Autodesk Inventor part; units mm, degrees
ref_plane "YZ Plane" through (0, 0, 0) normal (1, 0, 0) x (0, 1, 0)
ref_plane "XZ Plane" through (0, 0, 0) normal (0, 1, 0) x (-1, 0, 0)
ref_plane "XY Plane" through (0, 0, 0) normal (0, 0, 1) x (1, 0, 0)
sketch "Sketch1" plane through (0, 0, 0) normal (0, 0, 1) x (1, 0, 0)
  line L0 (21.4217, 22.24) -> (21.4217, 19.24)
  line L1 (21.4217, 22.24) -> (37.8228, 22.24)
  line L2 (21.4217, 19.24) -> (40.8228, 19.24)
  line L3 (40.8228, 27.84) -> (37.8228, 27.84)
  line L4 (37.8228, 27.84) -> (37.8228, 22.24)
  line L5 (40.8228, 27.84) -> (40.8228, 19.24)
  point P0 (0, 0)
extrude "Extrusion1" add sketch "Sketch1" along normal blind 40
sketch "Sketch2" plane through (40.8228, 19.24, 0) normal (1, 0, 0) x (0, 0, -1)
  line L0 (-40, 8.6) -> (-40, 0)
  line L1 (0, 8.6) -> (-40, 8.6)
  circle A0 centre (-37, 5.8) radius 1.35
  circle A1 centre (-20, 5.8) radius 1.35
  circle A2 centre (-3, 5.8) radius 1.35
  point P0 (0, -19.24)
  dimension "d2" = 2.7
  dimension "d3" = 2.7
  dimension "d4" = 2.8
  dimension "d5" = 2.8
  dimension "d6" = 17
  dimension "d7" = 2.7
  dimension "d8" = 17
  dimension "d9" = 3
extrude "Extrusion2" cut sketch "Sketch2" against normal through all
sketch "Sketch3" plane through (21.4217, 22.24, 0) normal (0, 1, 0) x (1, 0, 0)
  line L0 (16.4011, 0) -> (0, 0)
  line L1 (0, 0) -> (0, -40)
  circle A0 centre (2.8, -3) radius 1.35
  circle A1 centre (2.8, -20) radius 1.35
  circle A2 centre (2.8, -37) radius 1.35
  point P0 (-21.4217, 0)
  dimension "d12" = 2.7
  dimension "d13" = 3
  dimension "d14" = 2.8
  dimension "d15" = 2.7
  dimension "d16" = 2.7
  dimension "d17" = 17
  dimension "d18" = 17
extrude "Extrusion3" cut sketch "Sketch3" against normal through all
properties part number "Groin" material "Aluminum-6061"
Work out the finished part from the listing and answer in its coordinate system (mm). Give positions to 0.01 mm unless a question says otherwise; leave off trailing zeros. Loops run counter-clockwise (first coordinate to the right, second up) from the corner with the lowest first, then second, coordinate; pieces in that order, holes last. Notation, with made-up numbers: (49.25, -8) - (85.25, -8) arc R14 ccw to (85.25, 17) - close; hole circle Ø7 at (46.25, 65.5). An arc over 180 degrees is marked (long way). One line per question, with ' | ' between items.
(1) Each of these flat-tipped pins is pushed along its axis until it touches: pin 1 Ø8 at (x, z) = (30, 17) entering from +Y; pin 2 Ø1.7 at (y, z) = (25, 22) entering from -X. Where does it stop, or does it pass through?
Recorded:
pin 1: stops at y = 22.24 | pin 2: stops at x = 37.82
(2) The part is cut by section C-C (y = 25.04). Write down the section's boundary in (x, z), then the cut area to 3 significant figures.
Recorded:
outline: (37.82, 0) - (40.82, 0) - (40.82, 1.65) - (37.82, 1.65) - close; (37.82, 4.35) - (40.82, 4.35) - (40.82, 18.65) - (37.82, 18.65) - close; (37.82, 21.35) - (40.82, 21.35) - (40.82, 35.65) - (37.82, 35.65) - close; (37.82, 38.35) - (40.82, 38.35) - (40.82, 40) - (37.82, 40) - close | area: 95.7 mm²
(3) Straight lines are drawn through the part: probe 1 along X at (y, z) = (19.95, 20); probe 2 along Y at (x, z) = (39.8, 20); probe 3 along X at (y, z) = (25, 11.5). For each, find the intervals that lie inside material, in ascending order.
Recorded:
probe 1: x = 21.42 to 22.87, 25.57 to 40.82 | probe 2: y = 19.24 to 23.69, 26.39 to 27.84 | probe 3: x = 37.82 to 40.82
(4) The part is cut by section B-B (y = 20). Write down the section's boundary in (x, z), then the cut area to 3 significant figures.
Recorded:
outline: (21.42, 0) - (40.82, 0) - (40.82, 40) - (21.42, 40) - close; hole circle Ø2.7 at (24.22, 3); hole circle Ø2.7 at (24.22, 20); hole circle Ø2.7 at (24.22, 37) | area: 759 mm²
(5) The part is cut by section A-A (z = 20). Write down the section's boundary in (x, y).
Recorded:
outline: (21.42, 19.24) - (22.87, 19.24) - (22.87, 22.24) - (21.42, 22.24) - close; (25.57, 19.24) - (40.82, 19.24) - (40.82, 23.69) - (37.82, 23.69) - (37.82, 22.24) - (25.57, 22.24) - close; (37.82, 26.39) - (40.82, 26.39) - (40.82, 27.84) - (37.82, 27.84) - close
(6) The mould has two halves that part along X. Classify faces 1 (the face through (37.823, 27, 20)), 2 (the face through (24.84, 20.76, 38.2)), 3 (the face through (40.823, 23, 20)), 4 (the face through (30, 22.24, 20)): +X half, -X half, draft (parallel to the pull), parting line (faces both ways), or undercut.
Recorded:
face 1: -X half | face 2: undercut | face 3: +X half | face 4: draft
(7) The part is cut by section D-D (z = 16). Write down the section's boundary in (x, y).
Recorded:
outline: (21.42, 19.24) - (40.82, 19.24) - (40.82, 27.84) - (37.82, 27.84) - (37.82, 22.24) - (21.42, 22.24) - close
